Build history of the part. All positions in model axes, mm. Face numbers are marked on the shaded views. Give positions to 0.01 mm unless a question says otherwise; leave off trailing zeros. Loops run counter-clockwise (first coordinate to the right, second up) from the corner with the lowest first, then second, coordinate; pieces in that order, holes last.
1) Band-saw the part on C-C on x = -16. List the corners of the cut face in (y, z) (3 decimals), then the cut area to 3 significant figures.
2) Band-saw the part on B-B on y = 2.25. List the corners of the cut face in (x, z) (3 decimals), then the cut area to 3 significant figures.
3) Two-plate mould, pull along X, no slides. Class the marked faces 1, 2 and 3: +X half, -X half, draft (parallel to the pull), parting line (faces both ways), or undercut.
4) Band-saw the part on A-A on z = -7.5. List the corners of the cut face in (x, y) (3 decimals), then the cut area to 3 significant figures.
5) Wall check: line 1 (X direction, y = 3, z = -7) (3 decimals); line 2 (Z direction, x = -8, y = 6.25) (3 decimals); line 3 (X direction, y = 4, z = -26). Give the ranges that are in metal, low to high.
```python
from build123d import *

# Parameters (mm, degrees)
BOSS_EXTRUDE3_DEPTH = 6.35
SKETCH5_R           = 1.4224
SKETCH5_R_2         = 1.4732
CUT_EXTRUDE2_DEPTH  = 55.454774814


with BuildPart() as part:
    # Sketch2 → Boss-Extrude3 (new body)
    with BuildSketch(Plane(origin=(0, 0, 0), x_dir=(1, 0, 0), z_dir=(0, 1, 0))):
        with BuildLine():
            Line((-45, 25.825), (-45, -25.825))
            ThreePointArc((-45, -25.825), (-43.777170811, -28.777170811), (-40.825, -30))
            Line((-40.825, -30), (40.825, -30))
            ThreePointArc((40.825, -30), (43.777170811, -28.777170811), (45, -25.825))
            Line((45, -25.825), (45, 25.825))
            ThreePointArc((45, 25.825), (43.777170811, 28.777170811), (40.825, 30))
            Line((40.825, 30), (-40.825, 30))
            ThreePointArc((-40.825, 30), (-43.777170811, 28.777170811), (-45, 25.825))
        make_face()
        with BuildLine():
            Line((-41.825, -25.825), (-41.825, 25.825))
            ThreePointArc((-41.825, 25.825), (-41.532106781, 26.532106781), (-40.825, 26.825))
            Line((-40.825, 26.825), (40.825, 26.825))
            ThreePointArc((40.825, 26.825), (41.532106781, 26.532106781), (41.825, 25.825))
            Line((41.825, 25.825), (41.825, -25.825))
            ThreePointArc((41.825, -25.825), (41.532106781, -26.532106781), (40.825, -26.825))
            Line((40.825, -26.825), (-40.825, -26.825))
            ThreePointArc((-40.825, -26.825), (-41.532106781, -26.532106781), (-41.825, -25.825))
        make_face(mode=Mode.SUBTRACT)
    extrude(amount=BOSS_EXTRUDE3_DEPTH)

    # Sketch5 → Cut-Extrude2 (cut, through all)
    with BuildSketch(Plane.XZ):
        with Locations((-40.825, 25.825)):
            Circle(SKETCH5_R)
        with Locations((40.825, 25.81487963)):
            Circle(SKETCH5_R_2)
        with Locations((40.825, -25.825)):
            Circle(SKETCH5_R_2)
        with Locations((-40.825, -25.81356336)):
            Circle(SKETCH5_R_2)
    extrude(amount=-CUT_EXTRUDE2_DEPTH, mode=Mode.SUBTRACT)


solid = part.part
```
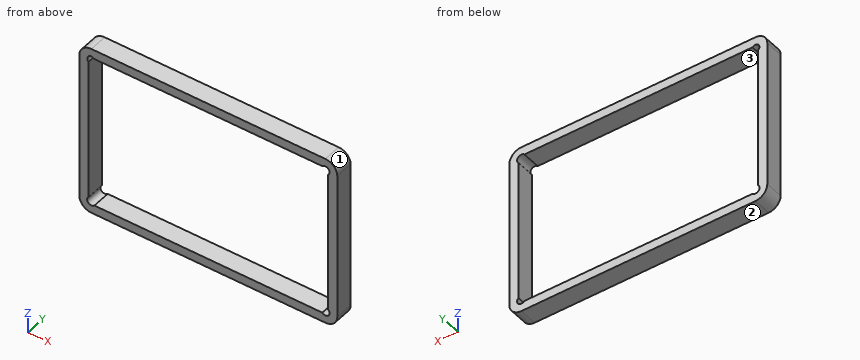
Findings below:
1. outline: (0, -30) - (6.35, -30) - (6.35, -26.825) - (0, -26.825) - close; (0, 26.825) - (6.35, 26.825) - (6.35, 30) - (0, 30) - close
1. area: 40.3 mm2
2. outline: (-45, -25.825) arc R4.175 ccw to (-40.825, -30) - (40.825, -30) arc R4.175 ccw to (45, -25.825) - (45, 25.825) arc R4.175 ccw to (40.825, 30) - (-40.825, 30) arc R4.175 ccw to (-45, 25.825) - close; hole (-41.825, -24.732) arc R1.473 ccw (long way) to (-39.754, -26.825) - (39.743, -26.825) arc R1.473 ccw (long way) to (41.825, -24.743) - (41.825, 24.733) arc R1.473 ccw (long way) to (39.753, 26.825) - (-39.813, 26.825) arc R1.422 ccw (long way) to (-41.825, 24.813) - close
2. area: 892 mm2
3. face 1: +X half
3. face 2: draft
3. face 3: undercut
4. outline: (-45, 0) - (-41.825, 0) - (-41.825, 6.35) - (-45, 6.35) - close; (41.825, 0) - (45, 0) - (45, 6.35) - (41.825, 6.35) - close
4. area: 40.3 mm2
5. line 1: x = -45 to -41.825, 41.825 to 45
5. line 2: z = -30 to -26.825, 26.825 to 30
5. line 3: x = -45 to -42.29, 42.29 to 45
